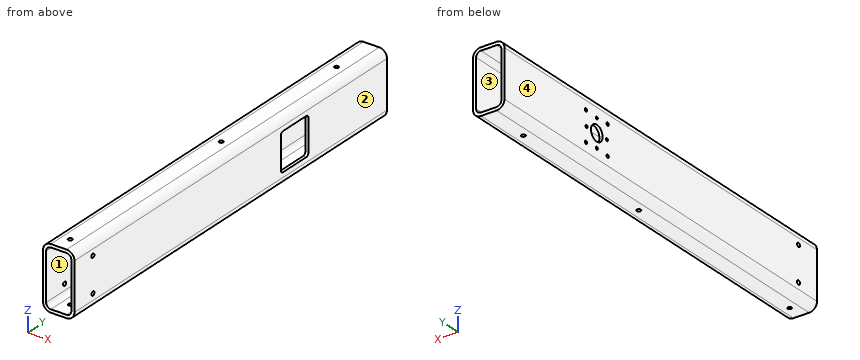
from build123d import *

# Parameters (mm, degrees)
RHS_C350_AS_100X50X5_0_RHS_C350_1_DEPTH = 677
SKETCH12_R                              = 2.25
CUT_EXTRUDE1_DEPTH                      = 10
CUT_EXTRUDE2_DEPTH                      = 10
SKETCH17_R                              = 12.5
SKETCH17_R_2                            = 2.5
CUT_EXTRUDE3_DEPTH                      = 10
SKETCH18_R                              = 3.25
CUT_EXTRUDE4_DEPTH                      = 354.846364966
SKETCH19_R                              = 3.25
CUT_EXTRUDE5_DEPTH                      = 354.846364966
SKETCH20_R                              = 3.25
CUT_EXTRUDE6_DEPTH                      = 346.806665638
SKETCH21_R                              = 2.25
CUT_EXTRUDE7_DEPTH                      = 10


with BuildPart() as part:
    # Sketch11 → Rhs c350 as 100X50X5.0 RHS C350(1) (new body)
    with BuildSketch(Plane(origin=(0, -338.5, 0), x_dir=(-1, 0, 0), z_dir=(0, 1, 0))):
        with BuildLine():
            Line((-12.5, -50), (12.5, -50))
            ThreePointArc((12.5, -50), (21.338834765, -46.338834765), (25, -37.5))
            Line((25, -37.5), (25, 37.5))
            ThreePointArc((25, 37.5), (21.338834765, 46.338834765), (12.5, 50))
            Line((12.5, 50), (-12.5, 50))
            ThreePointArc((-12.5, 50), (-21.338834765, 46.338834765), (-25, 37.5))
            Line((-25, 37.5), (-25, -37.5))
            ThreePointArc((-25, -37.5), (-21.338834765, -46.338834765), (-12.5, -50))
        make_face()
        with BuildLine():
            Line((-12.5, 45), (12.5, 45))
            ThreePointArc((12.5, 45), (17.803300859, 42.803300859), (20, 37.5))
            Line((20, 37.5), (20, -37.5))
            ThreePointArc((20, -37.5), (17.803300859, -42.803300859), (12.5, -45))
            Line((12.5, -45), (-12.5, -45))
            ThreePointArc((-12.5, -45), (-17.803300859, -42.803300859), (-20, -37.5))
            Line((-20, -37.5), (-20, 37.5))
            ThreePointArc((-20, 37.5), (-17.803300859, 42.803300859), (-12.5, 45))
        make_face(mode=Mode.SUBTRACT)
    extrude(amount=RHS_C350_AS_100X50X5_0_RHS_C350_1_DEPTH)

    # Sketch12 → Cut-Extrude1 (cut)
    with BuildSketch(Plane(origin=(25, 0, 0), x_dir=(0, 0, -1), z_dir=(1, 0, 0))):
        with Locations(Location((14.849242405, 153.349242405, 0), (0, 0, 90))):
            Circle(SKETCH12_R)
        with Locations(Location((-14.849242405, 153.349242405, 0), (0, 0, 90))):
            Circle(SKETCH12_R)
        with Locations(Location((-14.849242405, 123.650757595, 0), (0, 0, 90))):
            Circle(SKETCH12_R)
        with Locations(Location((14.849242405, 123.650757595, 0), (0, 0, 90))):
            Circle(SKETCH12_R)
    extrude(amount=-CUT_EXTRUDE1_DEPTH, mode=Mode.SUBTRACT)

    # Sketch16 → Cut-Extrude2 (cut)
    with BuildSketch(Plane(origin=(25, 0, 0), x_dir=(0, 0, -1), z_dir=(1, 0, 0))):
        with BuildLine():
            Line((-25, 108.5), (25, 108.5))
            ThreePointArc((25, 108.5), (28.535533906, 109.964466094), (30, 113.5))
            Line((30, 113.5), (30, 163.5))
            ThreePointArc((30, 163.5), (28.535533906, 167.035533906), (25, 168.5))
            Line((25, 168.5), (-25, 168.5))
            ThreePointArc((-25, 168.5), (-28.535533906, 167.035533906), (-30, 163.5))
            Line((-30, 163.5), (-30, 113.5))
            ThreePointArc((-30, 113.5), (-28.535533906, 109.964466094), (-25, 108.5))
        make_face()
    extrude(amount=-CUT_EXTRUDE2_DEPTH, mode=Mode.SUBTRACT)

    # Sketch17 → Cut-Extrude3 (cut)
    with BuildSketch(Plane(origin=(-20, 0, 0), x_dir=(0, 0, -1), z_dir=(1, 0, 0))):
        with Locations(Location((0, 138.5, 0), (0, 0, 90))):
            Circle(SKETCH17_R)
        with Locations(Location((-23.5, 162, 0), (0, 0, 90))):
            Circle(SKETCH17_R_2)
        with Locations(Location((23.5, 162, 0), (0, 0, 90))):
            Circle(SKETCH17_R_2)
        with Locations(Location((-23.5, 115, 0), (0, 0, 90))):
            Circle(SKETCH17_R_2)
        with Locations(Location((23.5, 115, 0), (0, 0, 90))):
            Circle(SKETCH17_R_2)
    extrude(amount=-CUT_EXTRUDE3_DEPTH, mode=Mode.SUBTRACT)

    # Sketch18 → Cut-Extrude4 (cut, through all)
    with BuildSketch(Plane(origin=(0, 0, -50), x_dir=(-1, 0, 0), z_dir=(0, 0, -1))):
        with Locations((0, 263.5)):
            Circle(SKETCH18_R)
        with Locations((0, 13.5)):
            Circle(SKETCH18_R)
    extrude(amount=-CUT_EXTRUDE4_DEPTH, mode=Mode.SUBTRACT)

    # Sketch19 → Cut-Extrude5 (cut, through all)
    with BuildSketch(Plane(origin=(0, 0, -50), x_dir=(-1, 0, 0), z_dir=(0, 0, -1))):
        with Locations((0, -313.5)):
            Circle(SKETCH19_R)
    extrude(amount=-CUT_EXTRUDE5_DEPTH, mode=Mode.SUBTRACT)

    # Sketch20 → Cut-Extrude6 (cut, through all)
    with BuildSketch(Plane(origin=(25, 0, 0), x_dir=(0, 0, -1), z_dir=(1, 0, 0))):
        with Locations(Location((27.5, -298.5, 0), (0, 0, 90))):
            Circle(SKETCH20_R)
        with Locations(Location((-27.5, -298.5, 0), (0, 0, 90))):
            Circle(SKETCH20_R)
    extrude(amount=-CUT_EXTRUDE6_DEPTH, mode=Mode.SUBTRACT)

    # Sketch21 → Cut-Extrude7 (cut)
    with BuildSketch(Plane(origin=(-20, 0, 0), x_dir=(0, 0, -1), z_dir=(1, 0, 0))):
        with Locations(Location((0, 160.5, 0), (0, 0, 90))):
            Circle(SKETCH21_R)
        with Locations(Location((22, 138.5, 0), (0, 0, 90))):
            Circle(SKETCH21_R)
        with Locations(Location((0, 116.5, 0), (0, 0, 90))):
            Circle(SKETCH21_R)
        with Locations(Location((-22, 138.5, 0), (0, 0, 90))):
            Circle(SKETCH21_R)
    extrude(amount=-CUT_EXTRUDE7_DEPTH, mode=Mode.SUBTRACT)


solid = part.part
Input: part model. Units: mm. Frame: model coordinates. Face numbers are marked on the shaded views. A direction names the side the tool comes from. Coordinates: 2 decimals unless noted, no trailing zeros.
(1) First-contact query: pin 1 Ø7.5 at (x, y) = (0, 263.5) entering from -Z; pin 2 Ø6 at (y, z) = (-298.5, -27.5) entering from +X; pin 3 Ø8 at (y, z) = (115, 23.5) entering from +X; pin 4 Ø2 at (x, y) = (18.5, -240.5) entering from -Z. Flat tips, straight axial feed; report the tip coordinate or a pass-through.
(2) Pull-direction query (Z, two-part tool) for the marked faces 1 and 2; classes: released by +Z, released by -Z, zero draft, split by the parting line, or undercut.
(3) Set-up query: the marked faces 3 and 4. Return all of +Z, -Z, +X, -X, +Y, -Y with unobstructed straight access to the full face (end or side cutting, diameter ignored); none if empty.
(4) Material intervals for probe 1 along Y at (x, z) = (0, -47); probe 2 along Z at (x, y) = (-12.5, 5); probe 3 along X at (y, z) = (103, 18), sorted ascending.
Data:
1. pin 1: stops at z = -50
1. pin 2: passes through
1. pin 3: stops at x = -20
1. pin 4: stops at z = -48.96
2. face 1: undercut
2. face 2: zero draft
3. face 3: +Y, -Y
3. face 4: +Z, -Z, -X, +Y, -Y
4. probe 1: y = -338.5 to -316.75, -310.25 to 10.25, 16.75 to 260.25, 266.75 to 338.5
4. probe 2: z = -50 to -45, 45 to 50
4. probe 3: x = -25 to -20, 20 to 25
